Check sheet for the modelled part. Datum: model origin and axes. Units: mm. A direction names the side the tool comes from. Coordinates: 2 decimals unless noted, no trailing zeros. Loops run counter-clockwise (first coordinate to the right, second up) from the corner with the lowest first, then second, coordinate; pieces in that order, holes last. Notation, with made-up numbers: (18, -25) - (72, -25) arc R17 cw to (72, 1) - close; hole circle Ø9 at (41.25, -25.5). An arc over 180 degrees is marked (long way). Use a Markdown table: item, result. Add a question column.
1) Tool access check on faces 1 (the flat face through (-3, -14, 5)), 2 (the flat face through (2.5, -16, 75)), 3 (the flat face through (-13.753, 15, 28)). Record the directions out of +Z, -Z, +X, -X, +Y, -Y that give a thin tool (end or side, any length) a straight path to the whole face; none if there is none.
2) Thickness scan on line 1 (Z direction, x = 11.5, y = -10); line 2 (Y direction, x = 0, z = 76.3); line 3 (Z direction, x = -5, y = -12.5). Record the ranges inside material, lowest first.
3) Sectioned sample at B-B, the plane x = 0. Enter the section's corners in (y, z), then the cut area to 3 significant figures.
4) Sectioned sample at C-C, the plane y = -5. Enter the section's corners in (x, z), then the cut area to 3 significant figures.
5) Sectioned sample at D-D, the plane z = 21. Enter the section's corners in (x, y).
6) Draft check along X on faces 4 (the cylindrical face through (12.543, -3.95, 68.549)), 5 (the flat face through (-4, -23.753, 2)), 6 (the cylindrical face through (-15.584, 0.526, 2.465)), 7 (the cylindrical face through (8.67, -15.2, 74.54)). Enter one of: pulls with the +X half, pulls with the -X half, needs draft (parallel to the pull), parting line crosses it, or undercut.
7) Sectioned sample at A-A, the plane z = 70. Enter the section's corners in (x, y), then the cut area to 3 significant figures.
8) Go/stop test with flat-tipped pins: P1, Ø12, axis at x = 11.5, z = 19, coming from the -Y side; P2, Ø2.5, axis at y = -3.5, z = 75.5, coming from the -X side; P3, Ø18, axis at x = -5, y = -5, coming from the -Z side; P4, Ø11.5, axis at x = -4.5, y = 0, coming from the +Z side. Record where each tip stops, or that it passes through.
from build123d import *

# Parameters (mm, degrees)
SKETCH1_R           = 1.75
BOSS_EXTRUDE1_DEPTH = 5
SKETCH2_R           = 1.35
BOSS_EXTRUDE2_DEPTH = 4
SKETCH4_W           = 7
SKETCH4_H           = 5
BOSS_EXTRUDE3_DEPTH = 72
SKETCH5_R           = 10
BOSS_EXTRUDE4_DEPTH = 5
SKETCH6_R           = 13.15
SKETCH6_R_2         = 11.15
BOSS_EXTRUDE5_DEPTH = 7
CUT_EXTRUDE1_START  = -3
SKETCH7_R           = 11.15
CUT_EXTRUDE1_DEPTH  = 3
CUT_EXTRUDE2_DEPTH  = 5


with BuildPart() as part:
    # Sketch1 → Boss-Extrude1 (new body)
    with BuildSketch(Plane.XY):
        with BuildLine():
            Line((-13.753194099, 0), (-13.753194099, 19.75))
            Line((-13.753194099, 19.75), (-20.753194099, 19.75))
            Line((-20.753194099, 19.75), (-20.753194099, 0))
            ThreePointArc((-20.753194099, 0), (-16.34718685, -12.785325472), (-5, -20.141873431))
            Line((-5, -20.141873431), (-5, -23.753194099))
            Line((-5, -23.753194099), (-2.5, -23.753194099))
            Line((-2.5, -23.753194099), (-2.5, -16.753194099))
            Line((-2.5, -16.753194099), (2.5, -16.753194099))
            Line((2.5, -16.753194099), (2.5, -23.753194099))
            Line((2.5, -23.753194099), (5, -23.753194099))
            Line((5, -23.753194099), (5, -20.141873431))
            ThreePointArc((5, -20.141873431), (16.34718685, -12.785325472), (20.753194099, 0))
            Line((20.753194099, 0), (20.753194099, 19.75))
            Line((20.753194099, 19.75), (13.753194099, 19.75))
            Line((13.753194099, 19.75), (13.753194099, 0))
            ThreePointArc((13.753194099, 0), (0, -13.753194099), (-13.753194099, 0))
        make_face()
        with Locations((-17.253194099, 0)):
            Circle(SKETCH1_R, mode=Mode.SUBTRACT)
        with Locations((-17.253194099, 10)):
            Circle(SKETCH1_R, mode=Mode.SUBTRACT)
        with Locations((17.253194099, 10)):
            Circle(SKETCH1_R, mode=Mode.SUBTRACT)
        with Locations((17.253194099, 0)):
            Circle(SKETCH1_R, mode=Mode.SUBTRACT)
    extrude(amount=BOSS_EXTRUDE1_DEPTH)

    # Sketch2 → Boss-Extrude2 (add)
    with BuildSketch(Plane(origin=(0, 0, 0), x_dir=(-1, 0, 0), z_dir=(0, 0, -1))):
        with Locations(Location((-17.253194099, 16.75, 0), (0, 0, 180))):
            Circle(SKETCH2_R)
        with Locations(Location((17.253194099, 16.75, 0), (0, 0, 180))):
            Circle(SKETCH2_R)
    extrude(amount=BOSS_EXTRUDE2_DEPTH)

    # Sketch4 → Boss-Extrude3 (add)
    with BuildSketch(Plane.XY.offset(5)):
        with Locations((-17.253194099, 17.25)):
            Rectangle(SKETCH4_W, SKETCH4_H)
        with Locations((17.253194099, 17.25)):
            Rectangle(SKETCH4_W, SKETCH4_H)
    extrude(amount=BOSS_EXTRUDE3_DEPTH)

    # Sketch5 → Boss-Extrude4 (add)
    with BuildSketch(Plane.XY.offset(77)):
        with BuildLine():
            Line((-13.753194099, 19.75), (-13.753194099, 14.75))
            Line((-13.753194099, 14.75), (-13.753194099, -10.821259264))
            ThreePointArc((-13.753194099, -10.821259264), (0, -17.5), (13.753194099, -10.821259264))
            Line((13.753194099, -10.821259264), (13.753194099, 14.75))
            Line((13.753194099, 14.75), (13.753194099, 19.75))
            Line((13.753194099, 19.75), (-13.753194099, 19.75))
        make_face()
        Circle(SKETCH5_R, mode=Mode.SUBTRACT)
    extrude(amount=-BOSS_EXTRUDE4_DEPTH)

    # Sketch6 → Boss-Extrude5 (add)
    with BuildSketch(Plane(origin=(0, 0, 72), x_dir=(-1, 0, 0), z_dir=(0, 0, -1))):
        with Locations(Location((0, 0, 0), (0, 0, 180))):
            Circle(SKETCH6_R)
        Circle(SKETCH6_R_2, mode=Mode.SUBTRACT)
    extrude(amount=BOSS_EXTRUDE5_DEPTH)

    # Sketch7 → Cut-Extrude1 (cut)
    with BuildSketch(Plane(origin=(0, 0, 72), x_dir=(-1, 0, 0), z_dir=(0, 0, -1)).offset(CUT_EXTRUDE1_START)):
        Circle(SKETCH7_R)
    extrude(amount=CUT_EXTRUDE1_DEPTH, mode=Mode.SUBTRACT)

    # Sketch8 → Cut-Extrude2 (cut)
    with BuildSketch(Plane.XY.offset(77)):
        with BuildLine():
            Line((2.5, -17.320508076), (2.5, -15))
            Line((2.5, -15), (-2.5, -15))
            Line((-2.5, -15), (-2.5, -17.320508076))
            ThreePointArc((-2.5, -17.320508076), (0, -17.5), (2.5, -17.320508076))
        make_face()
    extrude(amount=-CUT_EXTRUDE2_DEPTH, mode=Mode.SUBTRACT)


solid = part.part
Solved:
| question | item | result |
|---|---|---|
| 1 | face 1 | +X, -X, -Y |
| 1 | face 2 | +Z, -Y |
| 1 | face 3 | -Z, +Y |
| 2 | line 1 | z = 0 to 5, 72 to 77 |
| 2 | line 2 | y = -15 to -10, 10 to 19.75 |
| 2 | line 3 | z = 72 to 77 |
| 3 | outline | (-16.75, 0) - (-13.75, 0) - (-13.75, 5) - (-16.75, 5) - close; (-15, 72) - (-13.15, 72) - (-13.15, 65) - (-11.15, 65) - (-11.15, 75) - (-10, 75) - (-10, 77) - (-15, 77) - close; (10, 75) - (11.15, 75) - (11.15, 65) - (13.15, 65) - (13.15, 72) - (19.75, 72) - (19.75, 77) - (10, 77) - close |
| 3 | area | 110 mm2 |
| 4 | outline | (-20.14, 0) - (-12.81, 0) - (-12.81, 5) - (-20.14, 5) - close; (-13.75, 72) - (-12.16, 72) - (-12.16, 65) - (-9.97, 65) - (-9.97, 75) - (-8.66, 75) - (-8.66, 77) - (-13.75, 77) - close; (8.66, 75) - (9.97, 75) - (9.97, 65) - (12.16, 65) - (12.16, 72) - (13.75, 72) - (13.75, 77) - (8.66, 77) - close; (12.81, 0) - (20.14, 0) - (20.14, 5) - (12.81, 5) - close |
| 4 | area | 147 mm2 |
| 5 | outline | (-20.75, 14.75) - (-13.75, 14.75) - (-13.75, 19.75) - (-20.75, 19.75) - close; (13.75, 14.75) - (20.75, 14.75) - (20.75, 19.75) - (13.75, 19.75) - close |
| 6 | face 4 | parting line crosses it |
| 6 | face 5 | needs draft |
| 6 | face 6 | undercut |
| 6 | face 7 | pulls with the +X half |
| 7 | outline | (-20.75, 14.75) - (-13.75, 14.75) - (-13.75, 19.75) - (-20.75, 19.75) - close; circle Ø26.3 at (0, 0); (13.75, 14.75) - (20.75, 14.75) - (20.75, 19.75) - (13.75, 19.75) - close; hole circle Ø22.3 at (0, 0) |
| 7 | area | 223 mm2 |
| 8 | P1 | stops at y = 14.75 |
| 8 | P2 | stops at x = -13.75 |
| 8 | P3 | stops at z = 0 |
| 8 | P4 | stops at z = 77 |
